The model under review builds one solid part; all positions refer to its coordinate system, in mm. Round coordinates to 2 decimals unless told otherwise and drop trailing zeros. Order: outer loops, then holes, each group sorted by start corner. A loop starts at its lowest first (then second) coordinate and runs counter-clockwise, first axis right, second up. Notation, with made-up numbers: M -2.5,63 L 22.5,63 A35 cw 22.5,96 Z; hole C 8.5,41 d3. An arc over 180 degrees is marked long. Answer as a JSON object with one key per item and string values. Group by question number.
1) Consider section A-A, the plane x = 115. Write out the cut boundary in (y, z), then the cut area to 3 significant figures.
2) To check wall thickness, follow line 1 (Z direction, x = 203, y = 1.15); line 2 (X direction, y = 2.4, z = -70); line 3 (Z direction, x = 89, y = 1.45). State the ranges of each line that lie inside material, in increasing order.
3) Consider section B-B, the plane y = 1.7. Count the separate pieces of the cut face and the enclosed holes in it, then the cut area to 3 significant figures.
4) Consider section C-C, the plane z = -27.5. Write out the cut boundary in (x, y), then the cut area to 3 significant figures.
```python
from build123d import *

# Parameters (mm, degrees)
SKETCH_1_W           = 300
SKETCH_1_H           = 185
EXTRUDE_1_DEPTH      = 3
CUT_EXTRUDE_1_DEPTH  = 10
SKETCH_3_R           = 2.15
CUT_EXTRUDE_2_DEPTH  = 10
SKETCH_4_W           = 209.1
SKETCH_4_H           = 7
CUT_EXTRUDE_3_DEPTH  = 10
SKETCH_5_R           = 3.5
CUT_EXTRUDE_5_DEPTH  = 10
CHAMFER_1_SIZE       = 2.5
SKETCH_9_W           = 5
SKETCH_9_H           = 3
SKETCH_9_W_2         = 6
CUT_EXTRUDE_9_DEPTH  = 10
SKETCH_10_R          = 0.965981561
CUT_EXTRUDE_10_DEPTH = 10


with BuildPart() as part:
    # 스케치1 → 보스-돌출1 (new body)
    with BuildSketch(Plane(origin=(0, 0, 0), x_dir=(1, 0, 0), z_dir=(0, 1, 0))):
        with Locations((150, 92.5)):
            Rectangle(SKETCH_1_W, SKETCH_1_H)
    extrude(amount=EXTRUDE_1_DEPTH)

    # 스케치2 → 컷-돌출1 (cut)
    with BuildSketch(Plane(origin=(0, 3, 0), x_dir=(1, 0, 0), z_dir=(0, 1, 0))):
        Polygon((78.8, 61.106579113), (78.8, 86.106579113), (83.1, 86.106579113), (83.1, 36.106579113), (78.8, 36.106579113), align=None)
    extrude(amount=-CUT_EXTRUDE_1_DEPTH, mode=Mode.SUBTRACT)

    # 스케치3 → 컷-돌출2 (cut)
    with BuildSketch(Plane(origin=(0, 3, 0), x_dir=(1, 0, 0), z_dir=(0, 1, 0))):
        with Locations((80.95, 86.106579113)):
            Circle(SKETCH_3_R)
        with Locations((80.95, 36.106579113)):
            Circle(SKETCH_3_R)
    extrude(amount=-CUT_EXTRUDE_2_DEPTH, mode=Mode.SUBTRACT)

    # 스케치4 → 컷-돌출3 (cut)
    with BuildSketch(Plane(origin=(0, 3, 0), x_dir=(1, 0, 0), z_dir=(0, 1, 0))):
        with Locations((195.45, 157.5)):
            Rectangle(SKETCH_4_W, SKETCH_4_H)
        with Locations((195.45, 27.5)):
            Rectangle(SKETCH_4_W, SKETCH_4_H)
    extrude(amount=-CUT_EXTRUDE_3_DEPTH, mode=Mode.SUBTRACT)

    # 스케치5 → 컷-돌출5 (cut)
    with BuildSketch(Plane(origin=(0, 3, 0), x_dir=(1, 0, 0), z_dir=(0, 1, 0))):
        with Locations((90.9, 157.5)):
            Circle(SKETCH_5_R)
        with Locations((90.9, 27.5)):
            Circle(SKETCH_5_R)
    extrude(amount=-CUT_EXTRUDE_5_DEPTH, mode=Mode.SUBTRACT)

    # 모따기1
    chamfer_1_edges = [part.edges().sort_by_distance(p)[0] for p in [
        (0, 1.5, -185),
        (300, 1.5, -185),
        (300, 1.5, 0),
        (0, 1.5, 0),
    ]]
    chamfer(chamfer_1_edges, length=CHAMFER_1_SIZE)

    # 스케치9 → 컷-돌출9 (cut)
    with BuildSketch(Plane.XZ):
        with Locations((292.5, -175.5)):
            Rectangle(SKETCH_9_W, SKETCH_9_H)
        with Locations((43.7, -175.5)):
            Rectangle(SKETCH_9_W_2, SKETCH_9_H)
        with Locations((43.7, -9.5)):
            Rectangle(SKETCH_9_W_2, SKETCH_9_H)
        with Locations((292.5, -9.5)):
            Rectangle(SKETCH_9_W, SKETCH_9_H)
    extrude(amount=-CUT_EXTRUDE_9_DEPTH, mode=Mode.SUBTRACT)

    # 스케치10 → 컷-돌출10 (cut)
    with BuildSketch(Plane(origin=(0, 3, 0), x_dir=(1, 0, 0), z_dir=(0, 1, 0))):
        with Locations((294.034018439, 174)):
            Circle(SKETCH_10_R)
        with Locations((290.965981561, 174)):
            Circle(SKETCH_10_R)
        with Locations((290.965981561, 177)):
            Circle(SKETCH_10_R)
        with Locations((294.034018439, 177)):
            Circle(SKETCH_10_R)
        with Locations((41.665981561, 174)):
            Circle(SKETCH_10_R)
        with Locations((41.665981561, 177)):
            Circle(SKETCH_10_R)
        with Locations((45.734018439, 177)):
            Circle(SKETCH_10_R)
        with Locations((45.734018439, 174)):
            Circle(SKETCH_10_R)
        with Locations((45.734018439, 11)):
            Circle(SKETCH_10_R)
        with Locations((45.734018439, 8)):
            Circle(SKETCH_10_R)
        with Locations((41.665981561, 8)):
            Circle(SKETCH_10_R)
        with Locations((41.665981561, 11)):
            Circle(SKETCH_10_R)
        with Locations((294.034018439, 8)):
            Circle(SKETCH_10_R)
        with Locations((290.965981561, 8)):
            Circle(SKETCH_10_R)
        with Locations((290.965981561, 11)):
            Circle(SKETCH_10_R)
        with Locations((294.034018439, 11)):
            Circle(SKETCH_10_R)
    extrude(amount=-CUT_EXTRUDE_10_DEPTH, mode=Mode.SUBTRACT)


solid = part.part
```
Results list:
{
 "1": {"outline": "M 0,-185 L 3,-185 L 3,-161 L 0,-161 Z; M 0,-154 L 3,-154 L 3,-31 L 0,-31 Z; M 0,-24 L 3,-24 L 3,0 L 0,0 Z", "area": "513 mm^2"},
 "2": {"line 1": "-185 to -161, -154 to -31, -24 to 0", "line 2": "0 to 78.8, 83.1 to 300", "line 3": "-185 to -160.44, -154.56 to -30.44, -24.56 to 0"},
 "3": {"separate pieces": "1", "enclosed holes": "5", "area": "52,200 mm^2"},
 "4": {"outline": "M 0,0 L 87.4,0 L 87.4,3 L 0,3 Z", "area": "262 mm^2"}
}
